from build123d import *

# Parameters (mm, degrees)
BASEHEAD_DEPTH                      = 6.63
INDENT_OUTLINE_R                    = 7
INDENT_DEPTH                        = 0.82875
SKETCH4_W                           = 0.6
SKETCH4_H                           = 11.237604307
THDSCHPAT_COUNT                     = 19
THDSCHPAT_PITCH                     = 1.5
SKETCH7_R                           = 13.935804787
CUT_EXTRUDE1_DEPTH                  = 10
SKETCH8_R                           = 7
BOSS_EXTRUDE1_DEPTH                 = 265
SKETCH9_W                           = 14.54473127
SKETCH9_H                           = 2.205507465
CUT_EXTRUDE2_DEPTH                  = 170
CUT_EXTRUDE3_REACH                  = 260.56
CUT_EXTRUDE3_END_RADIUS             = 7
SKETCH10_R                          = 2.5
CUT_EXTRUDE3_DIRECTION_2_REACH      = 260.56
CUT_EXTRUDE3_DIRECTION_2_END_RADIUS = 7


# Read off the part's stored shape, not the designer's step: Indent
with BuildPart() as part:
    # Sketch1 → BaseHead (new body)
    with BuildSketch(Plane(origin=(0, 0, 0), x_dir=(0, 0, -1), z_dir=(1, 0, 0))):
        Polygon((8, 4.618802154), (8, -4.618802154), (0, -9.237604307), (-8, -4.618802154), (-8, 4.618802154), (0, 9.237604307), align=None)
    extrude(amount=BASEHEAD_DEPTH)

    # BodySke → BaseBody (revolve)
    with BuildSketch(Plane.XY, mode=Mode.PRIVATE) as basebody_sk:
        Polygon((0, 0), (36.63, 0), (36.63, 4.172), (35.802, 5), (0, 5), align=None)
    revolve(basebody_sk.sketch.rotate(Axis((0, 0, 0), (1, 0, 0)), 90), axis=Axis((0, 0, 0), (1, 0, 0)))

    # Indent outline → Indent (cut)
    with BuildSketch(Plane.YZ):
        with Locations((0.192376607, 0.033212245)):
            Circle(INDENT_OUTLINE_R)
    extrude(amount=INDENT_DEPTH, mode=Mode.SUBTRACT)

    # Sketch3 → HeadChamfer (revolve, cut)
    with BuildSketch(Plane.XY):
        Polygon((0, 8), (3.601282526, 14.237604307), (3.601282526, 19.237604307), (-10, 19.237604307), (-10, 8), align=None)
    revolve(axis=Axis((0, 0, 0), (1, 0, 0)), mode=Mode.SUBTRACT)

    # Sketch4 → BearingFace (revolve, cut)
    with BuildSketch(Plane.XY, mode=Mode.PRIVATE) as bearingface_sk:
        with Locations((6.33, 13.618802154)):
            Rectangle(SKETCH4_W, SKETCH4_H)
    revolve(bearingface_sk.sketch.rotate(Axis((0, 0, 0), (1, 0, 0)), 270), axis=Axis((0, 0, 0), (1, 0, 0)), mode=Mode.SUBTRACT)

    # ThdSchSke → ThreadSchematic (revolve, cut)
    with BuildSketch(Plane.XY):
        Polygon((8.13, -4.172), (7.550228158, -5), (7.550228158, -6.25), (8.709771842, -6.25), (8.709771842, -5), align=None)
    threadschematic = revolve(axis=Axis((-3.175, 0, 0), (1, 0, 0)), mode=Mode.SUBTRACT)

    # ThdSchPat: ThreadSchematic ×19
    with Locations(*[(i * THDSCHPAT_PITCH, 0, 0) for i in range(1, THDSCHPAT_COUNT)]):
        add(threadschematic, mode=Mode.SUBTRACT)

    # Sketch7 → Cut-Extrude1 (cut)
    with BuildSketch(Plane(origin=(6.63, 0, 0), x_dir=(0, 0, -1), z_dir=(1, 0, 0))):
        Circle(SKETCH7_R)
    extrude(amount=-CUT_EXTRUDE1_DEPTH, mode=Mode.SUBTRACT)

    # Sketch8 → Boss-Extrude1 (add)
    with BuildSketch(Plane.ZY.offset(-6.63)):
        Circle(SKETCH8_R)
    extrude(amount=BOSS_EXTRUDE1_DEPTH)

    # Sketch9 → Cut-Extrude2 (cut)
    with BuildSketch(Plane(origin=(6.63, 0, 0), x_dir=(0, 0, -1), z_dir=(1, 0, 0))):
        with Locations((-1.022041736, -6.802753733)):
            Rectangle(SKETCH9_W, SKETCH9_H)
        with Locations((-1.022041736, 6.802753733)):
            Rectangle(SKETCH9_W, SKETCH9_H)
    extrude(amount=-CUT_EXTRUDE2_DEPTH, mode=Mode.SUBTRACT)

    # Cut-Extrude3: up to this cylinder (the profile starts inside it)
    cut_extrude3_end = Plane(origin=(-250.87, 0, 0), z_dir=(1, 0, 0)) * Cylinder(CUT_EXTRUDE3_END_RADIUS, 536.12, mode=Mode.PRIVATE)
    # Sketch10 → Cut-Extrude3 (cut, up to the surface)
    with BuildSketch(Plane(origin=(0, 0, 0), x_dir=(1, 0, 0), z_dir=(0, 1, 0)), mode=Mode.PRIVATE) as cut_extrude3_sk1:
        with Locations(Location((-250.87, 0, 0), (0, 0, 90))):
            Circle(SKETCH10_R)
    cut_extrude3_tool1 = extrude(cut_extrude3_sk1.sketch, amount=-CUT_EXTRUDE3_REACH, mode=Mode.PRIVATE) & cut_extrude3_end
    add(cut_extrude3_tool1.solids().sort_by_distance((-250.87, 0, 0))[0], mode=Mode.SUBTRACT)

    # Cut-Extrude3 direction 2: up to this cylinder (the profile starts inside it)
    cut_extrude3_direction_2_end = Plane(origin=(-250.87, 0, 0), z_dir=(1, 0, 0)) * Cylinder(CUT_EXTRUDE3_DIRECTION_2_END_RADIUS, 536.12, mode=Mode.PRIVATE)
    # Sketch10 → Cut-Extrude3 direction 2 (cut, up to the surface)
    with BuildSketch(Plane(origin=(0, 0, 0), x_dir=(1, 0, 0), z_dir=(0, 1, 0)), mode=Mode.PRIVATE) as cut_extrude3_direction_2_sk1:
        with Locations(Location((-250.87, 0, 0), (0, 0, 90))):
            Circle(SKETCH10_R)
    cut_extrude3_direction_2_tool1 = extrude(cut_extrude3_direction_2_sk1.sketch, amount=CUT_EXTRUDE3_DIRECTION_2_REACH, mode=Mode.PRIVATE) & cut_extrude3_direction_2_end
    add(cut_extrude3_direction_2_tool1.solids().sort_by_distance((-250.87, 0, 0))[0], mode=Mode.SUBTRACT)


solid = part.part
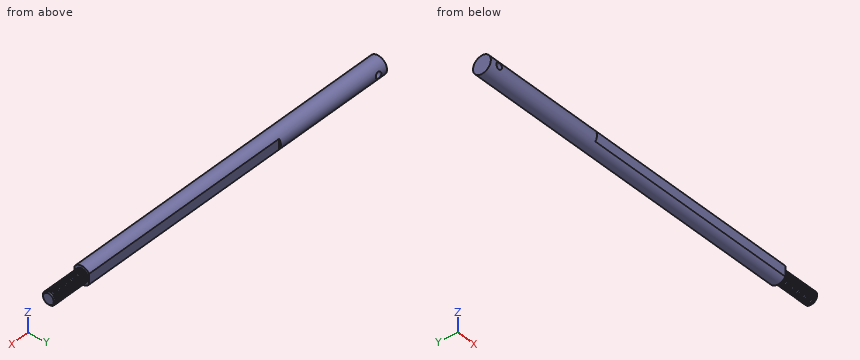
Read the model definition and answer for the solid it produces. Units are mm, in the model's axes. Give positions to 0.01 mm unless a question says otherwise; leave off trailing zeros. Loops run counter-clockwise (first coordinate to the right, second up) from the corner with the lowest first, then second, coordinate; pieces in that order, holes last. Notation, with made-up numbers: (9, 21.25) -> (45, 21.25) arc R30 cw to (45, 58.25) -> close; hole circle Ø3 at (24, 86). An arc over 180 degrees is marked (long way). Use a Markdown table: item, result.
Q1. Find the intervals of material crossed by line 1 along Z through (x, y) = (-250.87, 0.75); line 2 along X through (y, z) = (4, 0); line 3 along X through (y, z) = (-4.75, 4.25), in increasing order.
Solved:
| item | result |
|---|---|
| line 1 | z = -6.96 to -2.5, 2.5 to 6.96 |
| line 2 | x = -258.37 to -253.37, -248.37 to 36.63 |
| line 3 | x = -258.37 to 6.63 |
Q2. Each of these flat-tipped pins is pushed along its axis until it touches: pin 1 (2.5 mm diameter, centred on x = -71, z = -2, fed in from +Y); pin 2 (6.5 mm diameter, centred on x = -87.5, z = -1.5, fed in from -Y); pin 3 (3 mm diameter, centred on x = -203, z = -4, fed in from -Y). Where does it stop, or does it pass through?
Solved:
| item | result |
|---|---|
| pin 1 | stops at y = 5.7 |
| pin 2 | stops at y = -5.7 |
| pin 3 | stops at y = -6.54 |
Q3. Section B-B, the plane x = -6.5 is taken. Determine the outline of the cut face in (y, z), then the cut area to 3 significant figures.
Solved:
| item | result |
|---|---|
| outline | (-5.7, -4.06) arc R7 ccw to (5.7, -4.06) -> (5.7, 4.06) arc R7 ccw to (-5.7, 4.06) -> close |
| area | 140 mm^2 |
Q4. Section A-A, the plane x = -179 is taken. Determine the outline of the cut face in (y, z), then the cut area to 3 significant figures.
Solved:
| item | result |
|---|---|
| outline | circle Ø14 at (0, 0) |
| area | 154 mm^2 |
